from build123d import *

# Parameters (mm, degrees)
SZKIC1_W                    = 10
SZKIC1_H                    = 42
DODANIE_WYCI_GNI_CIE1_DEPTH = 1.5
ZAOKR_GLENIE1_R             = 2
SZKIC2_W                    = 1.5
SZKIC2_H                    = 38
DODANIE_WYCI_GNI_CIE2_DEPTH = 1
SZKIC3_W                    = 1.5
SZKIC3_H                    = 38
DODANIE_WYCI_GNI_CIE3_DEPTH = 1
SZKIC4_W                    = 6
SZKIC4_H                    = 1.5
DODANIE_WYCI_GNI_CIE4_DEPTH = 1
SZKIC5_W                    = 6
SZKIC5_H                    = 2
WYTNIJ_WYCI_GNI_CIE2_DEPTH  = 2.5


with BuildPart() as part:
    # Szkic1 → Dodanie-wyciągnięcie1 (new body)
    with BuildSketch(Plane.XY):
        with Locations((5, 21)):
            Rectangle(SZKIC1_W, SZKIC1_H)
    extrude(amount=DODANIE_WYCI_GNI_CIE1_DEPTH)

    # Zaokrąglenie1
    zaokr_glenie1_edges = [part.edges().sort_by_distance(p)[0] for p in [
        (0, 42, 0.75),
        (10, 42, 0.75),
        (10, 0, 0.75),
        (0, 0, 0.75),
    ]]
    fillet(zaokr_glenie1_edges, radius=ZAOKR_GLENIE1_R)

    # Szkic2 → Dodanie-wyciągnięcie2 (add)
    with BuildSketch(Plane(origin=(10, 0, 0), x_dir=(0, 0, -1), z_dir=(1, 0, 0))):
        with Locations((-0.75, 21)):
            Rectangle(SZKIC2_W, SZKIC2_H)
    extrude(amount=DODANIE_WYCI_GNI_CIE2_DEPTH)

    # Szkic3 → Dodanie-wyciągnięcie3 (add)
    with BuildSketch(Plane.ZY):
        with Locations((0.75, 21)):
            Rectangle(SZKIC3_W, SZKIC3_H)
    extrude(amount=DODANIE_WYCI_GNI_CIE3_DEPTH)

    # Szkic4 → Dodanie-wyciągnięcie4 (add)
    with BuildSketch(Plane(origin=(0, 42, 0), x_dir=(1, 0, 0), z_dir=(0, 1, 0))):
        with Locations((5, -0.75)):
            Rectangle(SZKIC4_W, SZKIC4_H)
    extrude(amount=DODANIE_WYCI_GNI_CIE4_DEPTH)

    # Szkic5 → Wytnij-wyciągnięcie2 (cut, through all)
    with BuildSketch(Plane(origin=(0, 0, 0), x_dir=(-1, 0, 0), z_dir=(0, 0, -1))):
        with Locations((-5, 40)):
            Rectangle(SZKIC5_W, SZKIC5_H)
        with Locations((-5, 2)):
            Rectangle(SZKIC5_W, SZKIC5_H)
    extrude(amount=-WYTNIJ_WYCI_GNI_CIE2_DEPTH, mode=Mode.SUBTRACT)


solid = part.part
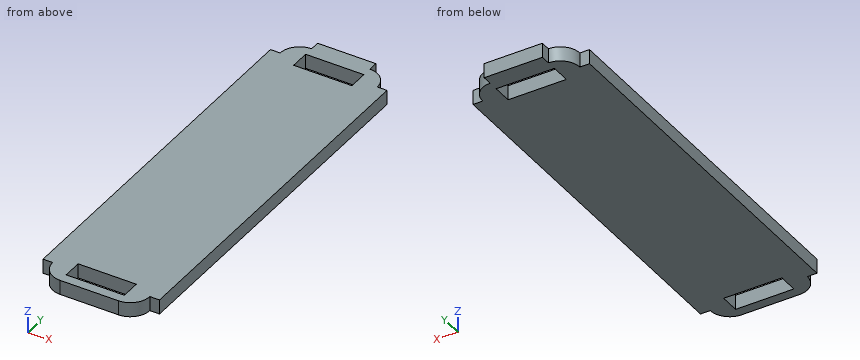
Verification items for the finished model (mm, model axes). Give positions to 0.01 mm unless a question says otherwise; leave off trailing zeros. Write each loop counter-clockwise with the first axis right and the second up, starting at its lowest first coordinate (ties: lowest second). Pieces come first, ordered by that corner, then holes.
(1) Cross-section at B-B (x = 3.25). Enter the section's corners in (y, z), plus the area to 3 significant figures.
(2) Cross-section at A-A (z = 1.2). Enter the section's corners in (x, y).
(3) Cross-section at C-C (x = 0.5). Enter the section's corners in (y, z), plus the area to 3 significant figures.
(4) Gauge pin test, flat ends, axial feed: pin 1 (0.8 mm diameter, centred on x = 10.5, z = 0.5, fed in from -Y); pin 2 (0.8 mm diameter, centred on x = 10.5, z = 1, fed in from +Y); pin 3 (0.8 mm diameter, centred on y = 42.5, z = 1, fed in from -X). Record the tip position at first contact, or that the pin passes through.
(5) Material ranges on line 1 (Y direction, x = 3.5, z = 1.15); line 2 (Y direction, x = 0.5, z = 1.3); line 3 (X direction, y = 41.5, z = 0.4), recorded low to high.
Worked out:
1. outline: (0, 0) - (1, 0) - (1, 1.5) - (0, 1.5) - close; (3, 0) - (39, 0) - (39, 1.5) - (3, 1.5) - close; (41, 0) - (43, 0) - (43, 1.5) - (41, 1.5) - close
1. area: 58.5 mm2
2. outline: (-1, 2) - (0, 2) arc R2 ccw to (2, 0) - (8, 0) arc R2 ccw to (10, 2) - (11, 2) - (11, 40) - (10, 40) arc R2 ccw to (8, 42) - (8, 43) - (2, 43) - (2, 42) arc R2 ccw to (0, 40) - (-1, 40) - close; hole (2, 1) - (8, 1) - (8, 3) - (2, 3) - close; hole (2, 39) - (8, 39) - (8, 41) - (2, 41) - close
3. outline: (0.68, 0) - (41.32, 0) - (41.32, 1.5) - (0.68, 1.5) - close
3. area: 61.0 mm2
4. pin 1: stops at y = 2
4. pin 2: stops at y = 40
4. pin 3: stops at x = 2
5. line 1: y = 0 to 1, 3 to 39, 41 to 43
5. line 2: y = 0.68 to 41.32
5. line 3: x = 0.68 to 9.32
